Could you check a few things on this model? Use its own coordinates, in mm. A direction names the side the tool comes from. Give positions to 0.01 mm unless a question says otherwise; leave off trailing zeros. Order: outer loops, then holes, each group sorted by start corner. A loop starts at its lowest first (then second) coordinate and runs counter-clockwise, first axis right, second up. Notation, with made-up numbers: (54.25, -40) -> (80.25, -40) arc R18 ccw to (80.25, -25) -> close; hole circle Ø8 at (-21, 72.5). An arc over 180 degrees is marked (long way). Write each question's results on one line, items separated by ' | '.
```python
from build123d import *

# Parameters (mm, degrees)
RESSALTO_EXTRUS_O1_DEPTH   = 34
RESSALTO_EXTRUS_O1_2_DEPTH = 34
RESSALTO_EXTRUS_O2_DEPTH   = 2
RESSALTO_EXTRUS_O3_START   = 34
RESSALTO_EXTRUS_O3_DEPTH   = 2
CORTE_EXTRUS_O1_REACH      = 194.531


with BuildPart() as part:
    # Esbo_o1 → Ressalto-extrus_o1 (new body)
    with BuildSketch(Plane.XY):
        Polygon((55.504617358, -134), (134, -55.504617358), (134, 55.504617358), (55.504617358, 134), (-55.504617358, 134), (-134, 55.504617358), (-134, -55.504617358), (-55.504617358, -134), align=None)
        Polygon((130, -53.847763109), (130, 53.847763109), (53.847763109, 130), (-53.847763109, 130), (-130, 53.847763109), (-130, -53.847763109), (-53.847763109, -130), (53.847763109, -130), align=None, mode=Mode.SUBTRACT)
    extrude(amount=RESSALTO_EXTRUS_O1_DEPTH)



with BuildPart() as body_2:
    # Esbo_o1 → Ressalto-extrus_o1 2 (new body)
    with BuildSketch(Plane.XY):
        Polygon((41.421356237, -100), (100, -41.421356237), (100, 41.421356237), (41.421356237, 100), (-41.421356237, 100), (-100, 41.421356237), (-100, -41.421356237), (-41.421356237, -100), align=None)
        Polygon((96, -39.764501988), (96, 39.764501988), (39.764501988, 96), (-39.764501988, 96), (-96, 39.764501988), (-96, -39.764501988), (-39.764501988, -96), (39.764501988, -96), align=None, mode=Mode.SUBTRACT)
    extrude(amount=RESSALTO_EXTRUS_O1_2_DEPTH)


with BuildPart() as part_1:
    add(part.part)

    add(body_2.part)  # Ressalto-extrus_o2 merges body 2
    # Esbo_o1_6 → Ressalto-extrus_o2 (add)
    with BuildSketch(Plane.XY):
        Polygon((53.847763109, -130), (130, -53.847763109), (130, 53.847763109), (53.847763109, 130), (-53.847763109, 130), (-130, 53.847763109), (-130, -53.847763109), (-53.847763109, -130), align=None)
        Polygon((100, -41.421356237), (100, 41.421356237), (41.421356237, 100), (-41.421356237, 100), (-100, 41.421356237), (-100, -41.421356237), (-41.421356237, -100), (41.421356237, -100), align=None, mode=Mode.SUBTRACT)
    extrude(amount=RESSALTO_EXTRUS_O2_DEPTH)

    # Esbo_o1_7 → Ressalto-extrus_o3 (add)
    with BuildSketch(Plane.XY.offset(RESSALTO_EXTRUS_O3_START)):
        Polygon((53.847763109, -130), (130, -53.847763109), (130, 53.847763109), (53.847763109, 130), (-53.847763109, 130), (-130, 53.847763109), (-130, -53.847763109), (-53.847763109, -130), align=None)
        Polygon((100, -41.421356237), (100, 41.421356237), (41.421356237, 100), (-41.421356237, 100), (-100, 41.421356237), (-100, -41.421356237), (-41.421356237, -100), (41.421356237, -100), align=None, mode=Mode.SUBTRACT)
    extrude(amount=-RESSALTO_EXTRUS_O3_DEPTH)

    # Esbo_o2 → Corte-extrus_o1 (cut, up to next)
    with BuildSketch(Plane.XY.offset(34), mode=Mode.PRIVATE) as corte_extrus_o1_sk1:
        Polygon((-134, -55.504617358), (-69.646752982, -119.857864376), (-53.906637612, -81.857864376), (-96, -39.764501988), (-96, 39.764501988), (-39.764501988, 96), (39.764501988, 96), (96, 39.764501988), (96, -39.764501988), (39.764501988, -96), (-19.764501988, -96), (-35.504617358, -134), (55.504617358, -134), (134, -55.504617358), (134, 55.504617358), (55.504617358, 134), (-55.504617358, 134), (-134, 55.504617358), align=None)
    corte_extrus_o1_tool1 = extrude(corte_extrus_o1_sk1.sketch, amount=-CORTE_EXTRUS_O1_REACH, mode=Mode.PRIVATE) & part_1.part
    add(corte_extrus_o1_tool1.solids().sort_by_distance((-99.143376, -85.001241, 34))[0], mode=Mode.SUBTRACT)


solid = part_1.part
```
Q1. I'm going to push flat-ended pins straight in: pin 1 Ø10 at (x, z) = (-28.5, 20) entering from -Y; pin 2 Ø1.5 at (y, z) = (-117.5, 16) entering from +X; pin 3 Ø6 at (x, z) = (-32, 13.5) entering from +Y; pin 4 Ø10 at (y, z) = (-96.5, 3.5) entering from +X. Where does each tip first touch, or does it pass through?
Here are the results:
pin 1: stops at y = -100 | pin 2: stops at x = -65.6 | pin 3: stops at y = -96 | pin 4: stops at x = -19.76
Q2. Suppose I cut it at B-B on x = -50.5. Please give me the cut outline in (y, z).
Here are the results:
outline: (-134, 0) -> (-85.26, 0) -> (-85.26, 34) -> (-134, 34) -> close; hole (-130, 2) -> (-90.92, 2) -> (-90.92, 32) -> (-130, 32) -> close
Q3. For faces 5 (the flat face through (-45, -113, 2)), 6 (the flat face through (-44, -130, 17)), 7 (the flat face through (-32, -100, 17)), which set-ups out of +Z, -Z, +X, -X, +Y, -Y let a thin tool reach every point of the face, with its end or its side?
Here are the results:
face 5: none | face 6: +X | face 7: +X, -X
Q4. Suppose I cut it at C-C on y = -109.5. Please give me the cut outline in (x, z).
Here are the results:
outline: (-65.36, 0) -> (-25.36, 0) -> (-25.36, 2) -> (-65.36, 2) -> close; (-65.36, 32) -> (-25.36, 32) -> (-25.36, 34) -> (-65.36, 34) -> close
Q5. I need wall thicknesses on line 1 along Z through (x, y) = (-43, -121.5); line 2 along Y through (x, z) = (-53, 13); line 3 along Y through (x, z) = (-55, 10). Which ranges of each line are inside material? Lowest first, please.
Here are the results:
line 1: z = 0 to 2, 32 to 34 | line 2: y = -134 to -130, -88.42 to -82.76 | line 3: y = -134 to -128.85, -86.42 to -84.5
Q6. Thinking about a two-plate mould opening in Z: for faces 1 (the flat face through (-30, -96, 17)), 2 (the flat face through (-45, -113, 0)), 3 (the flat face through (-45, -113, 34)), 4 (the flat face through (-48.59, -92.83, 16.79)), which applies, +Z half, -Z half, draft (parallel to the pull), parting line (faces both ways), or undercut?
Here are the results:
face 1: draft | face 2: -Z half | face 3: +Z half | face 4: undercut
Q7. Suppose I cut it at D-D on y = -89. Please give me the cut outline in (x, z) (1 decimal).
Here are the results:
outline: (-56.9, 0) -> (-46.8, 0) -> (-46.8, 34) -> (-56.9, 34) -> (-56.9, 32) -> (-52.4, 32) -> (-52.4, 2) -> (-56.9, 2) -> close
Q8. Suppose I cut it at A-A on z = 9.5. Please give me the cut outline in (x, y).
Here are the results:
outline: (-69.65, -119.86) -> (-55.5, -134) -> (-35.5, -134) -> (-33.85, -130) -> (-53.85, -130) -> (-67.99, -115.86) -> close; (-55.56, -85.86) -> (-41.42, -100) -> (-21.42, -100) -> (-19.76, -96) -> (-39.76, -96) -> (-53.91, -81.86) -> close
